Input: part model. Units: mm. Frame: model coordinates. A direction names the side the tool comes from. Round coordinates to 2 decimals unless told otherwise and drop trailing zeros. Order: outer loops, then holes, each group sorted by start corner. A loop starts at its lowest first (then second) coordinate and runs counter-clockwise, first axis right, second up.
Item 1: Cut plane A-A on x = 0. Output: boundary loops of the cut face in (y, z), then the cut area to 3 significant figures.
Item 2: Cut plane B-B on z = 0. Output: boundary loops of the cut face in (x, y).
Item 3: Mould query, pull axis Z, two halves, no side actions, for faces 1 (the cylindrical face through (-10.316, 36.538, -7.91)), 2 (the cylindrical face through (-3.47, 34.51, -15.62)), 3 (the flat face through (0, 0, 0)). Classes: released by +Z, released by -Z, zero draft, split by the parting line, or undercut.
Item 4: Reachability of faces 4 (the flat face through (0, 4, 0)), 5 (the flat face through (-1.3, 70, -13.1)) from +Z, -Z, +X, -X, +Y, -Y: full face, straight path, thin tool, end or side. Return the list, or none.
Item 5: Line query: L1, parallel to X at y = 54.5, z = 0; L2, parallel to Y at x = -4, z = 2.5. Output: solid intervals per line, ascending.
Item 6: Cut plane C-C on y = 11.5. Output: boundary loops of the cut face in (x, z).
Item 7: First-contact query: pin 1 (6 mm diameter, centred on x = -7, y = 35.5, fed in from +Z); pin 2 (8 mm diameter, centred on y = 53, z = 11, fed in from +X); pin 3 (1 mm diameter, centred on x = 2, y = 19.5, fed in from +Z). Flat tips, straight axial feed; report the tip coordinate or a pass-through.
Autodesk Fusion 360 part; units mm, degrees
sketch "Sketch1" plane through (0, 0, 0) normal (0, 1, 0) x (1, 0, 0)
  circle A0 centre (0, 0) radius 16
  circle A1 centre (0, 0) radius 13
  dimension "d1" = 32
  dimension "d7" = 3
extrude "Extrude1" add sketch "Sketch1" along normal blind 70 makes body 1
extrude "Extrude2" add sketch "Sketch1" along normal blind 4 contours A1 bodies 1
copy_body "Body->Comp1" bodies 1 removing the originals makes body 2 in component "tubeToolHolder04"
component "tubeToolHolder04" placed x (1, 0, 0) y (0, 1, 0) z (0, 0, 1) at (0, 0, 0)
From the geometry:
1. outline: (0, -16) - (70, -16) - (70, -13) - (4, -13) - (4, 13) - (70, 13) - (70, 16) - (0, 16) - close
1. area: 524 mm2
2. outline: (-16, 0) - (16, 0) - (16, 70) - (13, 70) - (13, 4) - (-13, 4) - (-13, 70) - (-16, 70) - close
3. face 1: undercut
3. face 2: split by the parting line
3. face 3: zero draft
4. face 4: +Y
4. face 5: +Z, -Z, +X, -X, +Y
5. L1: x = -16 to -13, 13 to 16
5. L2: y = 0 to 4
6. outline: circle Ø32 at (0, 0); hole circle Ø26 at (0, 0)
7. pin 1: stops at z = 15.49
7. pin 2: stops at x = 14.39
7. pin 3: stops at z = 15.93
